from build123d import *

# Parameters (mm, degrees)
ESQUISSE1_W           = 27
ESQUISSE1_H           = 6
BOSS_EXTRU_1_DEPTH    = 6
TROU_TARAUD_M31_D     = 2.5
TROU_TARAUD_M31_DEPTH = 8.5
TROU_TARAUD_M31_TIP   = 0.751075774
CHANFREIN1_SIZE       = 1.5
CHANFREIN1_SIZE2      = 3.533778549


with BuildPart() as part:
    # Esquisse1 → Boss.-Extru.1 (new body)
    with BuildSketch(Plane.XY):
        with Locations((13.5, -3)):
            Rectangle(ESQUISSE1_W, ESQUISSE1_H)
    extrude(amount=BOSS_EXTRU_1_DEPTH)

    # Trou taraudé M31
    with Locations(Plane(origin=(5, 0, 3), x_dir=(0, 0, 1), z_dir=(0, 1, 0))):
        with Locations((0, 0), (0, 17)):
            Hole(TROU_TARAUD_M31_D / 2, depth=TROU_TARAUD_M31_DEPTH)
            with Locations((0, 0, -(TROU_TARAUD_M31_DEPTH + TROU_TARAUD_M31_TIP / 2))):  # 118° drill point
                Cone(0, TROU_TARAUD_M31_D / 2, TROU_TARAUD_M31_TIP, mode=Mode.SUBTRACT)

    # Chanfrein1
    chanfrein1_edges = [part.edges().sort_by_distance(p)[0] for p in [
        (27, 0, 3),
    ]]
    chanfrein1_side = [part.faces().sort_by_distance(p)[0] for p in [
        (27, -3, 3),
    ]]
    chamfer(chanfrein1_edges, length=CHANFREIN1_SIZE, length2=CHANFREIN1_SIZE2, reference=chanfrein1_side[0])


solid = part.part
Input: part model. Units: mm. Frame: model coordinates. Round coordinates to 2 decimals unless told otherwise and drop trailing zeros. Loops run counter-clockwise (first coordinate to the right, second up) from the corner with the lowest first, then second, coordinate; pieces in that order, holes last. Notation, with made-up numbers: M 17,85 L 27,85 A28 ccw 27,120 Z; hole C 53,44 d5. An arc over 180 degrees is marked long. Answer as CSV lines item,"result". Start each with the question number.
(1) Section A-A, the plane x = 5. Output: boundary loops of the cut face in (y, z), plus the area to 3 significant figures.
(2) Line query: line 1 (X direction, y = -1.25, z = 3.9); line 2 (X direction, y = -5.25, z = 3.85); line 3 (Z direction, x = 5.75, y = -5.5). Output: solid intervals per line, ascending. Write a range as [from, to].
(3) Section B-B, the plane y = -5. Output: boundary loops of the cut face in (x, z), plus the area to 3 significant figures.
(4) Section C-C, the plane z = 3. Output: boundary loops of the cut face in (x, y), plus the area to 3 significant figures.
(5) Section D-D, the plane y = -1.25. Output: boundary loops of the cut face in (x, z), plus the area to 3 significant figures.
(6) Draft query along Z for faces 1 (the flat face through (12, 0, 3)), 2 (the flat face through (13, -3, 0)), 3 (the cylindrical face through (3.891, -3.042, 2.423)). Return one class per face: released by +Z, released by -Z, zero draft, split by the parting line, or undercut.
(7) First-contact query: pin 1 (2 mm diameter, centred on x = 5, z = 3, fed in from -Y). Flat tip, straight axial feed; report the tip coordinate or a pass-through.
Values found:
1,outline,"M -6,0 L 0,0 L 0,1.75 L -6,1.75 Z; M -6,4.25 L 0,4.25 L 0,6 L -6,6 Z"
1,area,"21.0 mm²"
2,line 1,"x = [0, 4.13], [5.87, 21.13], [22.87, 26.41]"
2,line 2,"x = [0, 4.08], [5.92, 21.08], [22.92, 27]"
2,line 3,"z = [0, 2], [4, 6]"
3,outline,"M 0,0 L 27,0 L 27,6 L 0,6 Z; hole C 5,3 d2.5; hole C 22,3 d2.5"
3,area,"152 mm²"
4,outline,"M 0,-6 L 3.75,-6 L 3.75,0 L 0,0 Z; M 6.25,-6 L 20.75,-6 L 20.75,0 L 6.25,0 Z; M 23.25,-6 L 27,-6 L 27,-1.5 L 23.47,0 L 23.25,0 Z"
4,area,"129 mm²"
5,outline,"M 0,0 L 26.41,0 L 26.41,6 L 0,6 Z; hole C 5,3 d2.5; hole C 22,3 d2.5"
5,area,"149 mm²"
6,face 1,"zero draft"
6,face 2,"released by -Z"
6,face 3,"undercut"
7,pin 1,"passes through"
